```python
from build123d import *

# Parameters (mm, degrees)
SKETCH_1_W          = 138.5
SKETCH_1_H          = 55
EXTRUDE_1_DEPTH     = 11
EXTRUDE_2_DEPTH     = 10
SKETCH_3_W          = 82
SKETCH_3_H          = 10
CUT_EXTRUDE_1_DEPTH = 2
SKETCH_4_W          = 82
SKETCH_4_H          = 35
CUT_EXTRUDE_2_DEPTH = 2
SKETCH_5_R          = 17.5
CUT_EXTRUDE_3_DEPTH = 152.351412283
HOLE_WIZARD_M5_1_D  = 4.2
SKETCH_9_R          = 4
CUT_EXTRUDE_5_DEPTH = 5
SKETCH_10_R         = 2.5
CUT_EXTRUDE_6_DEPTH = 156.667112776
HOLE_WIZARD_M5_2_D  = 4.2


with BuildPart() as part:
    # 스케치1 → 보스-돌출1 (new body)
    with BuildSketch(Plane(origin=(0, 0, 0), x_dir=(1, 0, 0), z_dir=(0, 1, 0))):
        with Locations((69.25, 27.5)):
            Rectangle(SKETCH_1_W, SKETCH_1_H)
    extrude(amount=EXTRUDE_1_DEPTH)

    # 스케치2 → 보스-돌출2 (add)
    with BuildSketch(Plane(origin=(0, 0, -45), x_dir=(-1, 0, 0), z_dir=(0, 0, -1))):
        Polygon((-138.5, 11), (-138.5, 50), (-81.5, 50), (-60, 11), align=None)
    extrude(amount=-EXTRUDE_2_DEPTH)

    # 스케치3 → 컷-돌출1 (cut)
    with BuildSketch(Plane(origin=(0, 11, 0), x_dir=(1, 0, 0), z_dir=(0, 1, 0))):
        with Locations((97.5, 50)):
            Rectangle(SKETCH_3_W, SKETCH_3_H)
    extrude(amount=-CUT_EXTRUDE_1_DEPTH, mode=Mode.SUBTRACT)

    # 스케치4 → 컷-돌출2 (cut)
    with BuildSketch(Plane(origin=(0, 11, 0), x_dir=(1, 0, 0), z_dir=(0, 1, 0))):
        with Locations((97.5, 17.5)):
            Rectangle(SKETCH_4_W, SKETCH_4_H)
    extrude(amount=-CUT_EXTRUDE_2_DEPTH, mode=Mode.SUBTRACT)

    # 스케치5 → 컷-돌출3 (cut, through all)
    with BuildSketch(Plane.XY.offset(-35)):
        with Locations((110, 27)):
            Circle(SKETCH_5_R)
    extrude(amount=-CUT_EXTRUDE_3_DEPTH, mode=Mode.SUBTRACT)

    # M5 나사 구멍1 (through all)
    with Locations(Plane.XY.offset(-35)):
        with Locations((90.5, 38.25), (129.5, 38.25), (129.5, 15.75), (90.5, 15.75)):
            Hole(HOLE_WIZARD_M5_1_D / 2)

    # 스케치9 → 컷-돌출5 (cut)
    with BuildSketch(Plane(origin=(0, 0, 0), x_dir=(1, 0, 0), z_dir=(0, 1, 0))):
        with Locations(Location((7.5, 37.5, 0), (0, 0, 270))):
            Circle(SKETCH_9_R)
        with Locations(Location((52.5, 37.5, 0), (0, 0, 270))):
            Circle(SKETCH_9_R)
        with Locations(Location((7.5, 17.5, 0), (0, 0, 270))):
            Circle(SKETCH_9_R)
        with Locations(Location((52.5, 17.5, 0), (0, 0, 270))):
            Circle(SKETCH_9_R)
    extrude(amount=CUT_EXTRUDE_5_DEPTH, mode=Mode.SUBTRACT)

    # 스케치10 → 컷-돌출6 (cut, through all)
    with BuildSketch(Plane.XZ.offset(-5)):
        with Locations(Location((52.5, -17.5, 0), (0, 0, 270))):
            Circle(SKETCH_10_R)
        with Locations(Location((52.5, -37.5, 0), (0, 0, 270))):
            Circle(SKETCH_10_R)
        with Locations(Location((7.5, -37.5, 0), (0, 0, 270))):
            Circle(SKETCH_10_R)
        with Locations(Location((7.5, -17.5, 0), (0, 0, 270))):
            Circle(SKETCH_10_R)
    extrude(amount=-CUT_EXTRUDE_6_DEPTH, mode=Mode.SUBTRACT)

    # M5 나사 구멍2 (through all)
    with Locations(Plane(origin=(0, 11, 0), x_dir=(1, 0, 0), z_dir=(0, 1, 0))):
        with Locations((10, 47.5), (50, 47.5), (10, 7.5), (50, 7.5), (30, 27.5)):
            Hole(HOLE_WIZARD_M5_2_D / 2)


solid = part.part
```
Here's how the part is built. I have some questions about the finished solid (model axes, mm). A direction names the side the tool comes from. Coordinates: 2 decimals unless noted, no trailing zeros. Order: outer loops, then holes, each group sorted by start corner. A loop starts at its lowest first (then second) coordinate and runs counter-clockwise, first axis right, second up.
1) Imagine slicing it at C-C on x = 115. List the corners of the cut face in (y, z) for me, and give its area (3 significant figures).
2) Will these pins go through, and if not, where does the flat tip stop? pin 1 (4.5 mm diameter, centred on x = 52.5, z = -17.5, fed in from -Y); pin 2 (5.5 mm diameter, centred on x = 129.5, y = 38.25, fed in from -Z); pin 3 (12 mm diameter, centred on x = 73, y = 41.5, fed in from +Z); pin 4 (4 mm diameter, centred on x = 53.5, z = -37.5, fed in from -Y).
3) Imagine slicing it at B-B on x = 129.5. List the corners of the cut face in (y, z) for me, and give its area (3 significant figures).
4) Which directions (+Z, -Z, +X, -X, +Y, -Y) give clear straight access to the entire face, cutting with the end or side of a thin tool? Please do faces 1 (the face through (6, 8, -15.5)), 2 (the face through (97, 9, -18)), 3 (the face through (48.951, 2.465, -35.654)).
5) Imagine slicing it at D-D on y = 38.25. List the corners of the cut face in (x, z) for me.
6) I need wall thicknesses on line 1 (X direction, y = 2, z = -17.5); line 2 (Y direction, x = 110, z = -39.5); line 3 (X direction, y = 3.5, z = -35). Which ranges of each line are inside material? Lowest first, please.
7) Imagine slicing it at A-A on z = -37.5. List the corners of the cut face in (x, y) for me, and give its area (3 significant figures).
8) We'd pull the mould along X, two halves only. Please class faces 4 (the face through (68, 5, -55)), 5 (the face through (0, 5, -27)), 6 (the face through (6.7, 5, -34.9)), 7 (the face through (10.46, 5.42, -45.45)): +X half, -X half, draft (parallel to the pull), parting line (faces both ways), or undercut.
Response values:
1. outline: (0, -55) - (9, -55) - (9, -45) - (10.23, -45) - (10.23, -35) - (9, -35) - (9, 0) - (0, 0) - close; (43.77, -45) - (50, -45) - (50, -35) - (43.77, -35) - close
1. area: 570 mm2
2. pin 1: passes through
2. pin 2: stops at z = -45
2. pin 3: stops at z = -35
2. pin 4: stops at y = 5
3. outline: (0, -55) - (9, -55) - (9, -45) - (13.65, -45) - (13.65, -35) - (9, -35) - (9, 0) - (0, 0) - close; (17.85, -45) - (36.15, -45) - (36.15, -35) - (17.85, -35) - close; (40.35, -45) - (50, -45) - (50, -35) - (40.35, -35) - close
3. area: 821 mm2
4. face 1: +Y, -Y
4. face 2: +Z, +X, +Y
4. face 3: -Y
5. outline: (75.02, -45) - (88.4, -45) - (88.4, -35) - (75.02, -35) - close; (92.6, -45) - (96.6, -45) - (96.6, -35) - (92.6, -35) - close; (123.4, -45) - (127.4, -45) - (127.4, -35) - (123.4, -35) - close; (131.6, -45) - (138.5, -45) - (138.5, -35) - (131.6, -35) - close
6. line 1: x = 0 to 3.5, 11.5 to 48.5, 56.5 to 138.5
6. line 2: y = 0 to 9.5, 44.5 to 50
6. line 3: x = 0 to 4.38, 10.62 to 49.38, 55.62 to 138.5
7. outline: (0, 0) - (3.5, 0) - (3.5, 5) - (5, 5) - (5, 11) - (0, 11) - close; (10, 5) - (11.5, 5) - (11.5, 0) - (48.5, 0) - (48.5, 5) - (50, 5) - (50, 11) - (10, 11) - close; (55, 5) - (56.5, 5) - (56.5, 0) - (138.5, 0) - (138.5, 50) - (81.5, 50) - (60, 11) - (55, 11) - close; hole circle Ø4.2 at (90.5, 15.75); hole circle Ø4.2 at (90.5, 38.25); hole circle Ø35 at (110, 27); hole circle Ø4.2 at (129.5, 15.75); hole circle Ø4.2 at (129.5, 38.25)
7. area: 3,010 mm2
8. face 4: draft
8. face 5: -X half
8. face 6: undercut
8. face 7: undercut
